from build123d import *

# Parameters (mm, degrees)
SKETCH_1_W          = 120
SKETCH_1_H          = 40
EXTRUDE_1_DEPTH     = 4.5
SKETCH_2_R          = 1.6
CUT_EXTRUDE_1_DEPTH = 127.571126249


with BuildPart() as part:
    # 草图1 → 凸台-拉伸1 (new body)
    with BuildSketch(Plane(origin=(0, 0, 0), x_dir=(1, 0, 0), z_dir=(0, 1, 0))):
        with Locations((60, 20)):
            Rectangle(SKETCH_1_W, SKETCH_1_H)
    extrude(amount=EXTRUDE_1_DEPTH)

    # 草图2 → 切除-拉伸1 (cut, through all)
    with BuildSketch(Plane.XZ):
        with Locations(Location((8, -7, 0), (0, 0, 270))):
            Circle(SKETCH_2_R)
        with Locations(Location((32, -33, 0), (0, 0, 270))):
            Circle(SKETCH_2_R)
        with Locations(Location((32, -7, 0), (0, 0, 270))):
            Circle(SKETCH_2_R)
        with Locations(Location((100, -33, 0), (0, 0, 270))):
            Circle(SKETCH_2_R)
        with Locations(Location((20, -33, 0), (0, 0, 270))):
            Circle(SKETCH_2_R)
        with Locations(Location((100, -7, 0), (0, 0, 270))):
            Circle(SKETCH_2_R)
        with Locations(Location((20, -7, 0), (0, 0, 270))):
            Circle(SKETCH_2_R)
        with Locations(Location((112, -33, 0), (0, 0, 270))):
            Circle(SKETCH_2_R)
        with Locations(Location((112, -7, 0), (0, 0, 270))):
            Circle(SKETCH_2_R)
        with Locations(Location((8, -33, 0), (0, 0, 270))):
            Circle(SKETCH_2_R)
        with Locations(Location((88, -33, 0), (0, 0, 270))):
            Circle(SKETCH_2_R)
        with Locations(Location((88, -7, 0), (0, 0, 270))):
            Circle(SKETCH_2_R)
        with BuildLine():
            Line((77, -15), (43, -15))
            ThreePointArc((43, -15), (36, -22), (43, -29))
            Line((43, -29), (77, -29))
            ThreePointArc((77, -29), (84, -22), (77, -15))
        make_face()
    extrude(amount=-CUT_EXTRUDE_1_DEPTH, mode=Mode.SUBTRACT)


solid = part.part
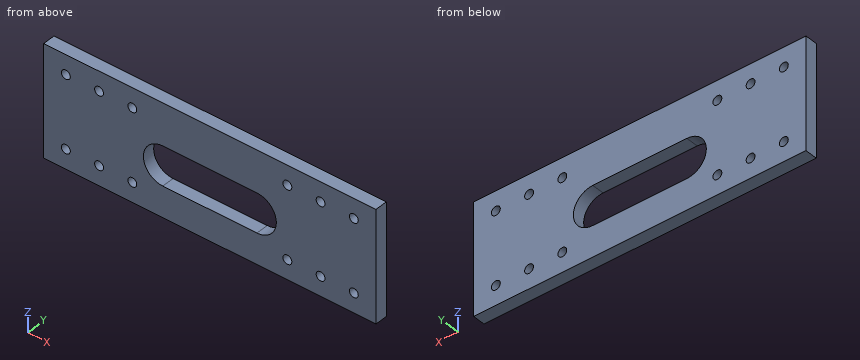
Geometry check sheet. Reference: the model listing, model coordinates, mm. Round coordinates to 2 decimals unless told otherwise and drop trailing zeros. Order: outer loops, then holes, each group sorted by start corner. A loop starts at its lowest first (then second) coordinate and runs counter-clockwise, first axis right, second up. Notation, with made-up numbers: M 15.5,-35.75 L 25.5,-35.75 A22 ccw 25.5,-13.75 Z; hole C 18.25,33.5 d4. An arc over 180 degrees is marked long. Answer in a Markdown table with one row per item. Add a question column.
Item 1: Sectioned sample at C-C, the plane x = 20. Enter the section's corners in (y, z), plus the area to 3 significant figures.
Item 2: Sectioned sample at B-B, the plane z = -33. Enter the section's corners in (x, y).
Item 3: Material ranges on L1, parallel to Z at x = 100, y = 1.3; L2, parallel to X at y = 0.9, z = -21.5; L3, parallel to Z at x = 47.5, y = 3.95, recorded low to high. Write a range as [from, to].
Item 4: Sectioned sample at A-A, the plane x = 68. Enter the section's corners in (y, z).
Item 5: Depth check by flat-ended pin: pin 1 Ø2.5 at (x, z) = (20, -7) entering from -Y. Enter the tip coordinate at first touch or a pass-through.
Item 6: Sectioned sample at D-D, the plane y = 1.2. State how many separate pieces and enclosed holes the cut face has, plus the area to 3 significant figures.
Filled in:
| question | item | result |
|---|---|---|
| 1 | outline | M 0,-40 L 4.5,-40 L 4.5,-34.6 L 0,-34.6 Z; M 0,-31.4 L 4.5,-31.4 L 4.5,-8.6 L 0,-8.6 Z; M 0,-5.4 L 4.5,-5.4 L 4.5,0 L 0,0 Z |
| 1 | area | 151 mm² |
| 2 | outline | M 0,0 L 6.4,0 L 6.4,4.5 L 0,4.5 Z; M 9.6,0 L 18.4,0 L 18.4,4.5 L 9.6,4.5 Z; M 21.6,0 L 30.4,0 L 30.4,4.5 L 21.6,4.5 Z; M 33.6,0 L 86.4,0 L 86.4,4.5 L 33.6,4.5 Z; M 89.6,0 L 98.4,0 L 98.4,4.5 L 89.6,4.5 Z; M 101.6,0 L 110.4,0 L 110.4,4.5 L 101.6,4.5 Z; M 113.6,0 L 120,0 L 120,4.5 L 113.6,4.5 Z |
| 3 | L1 | z = [-40, -34.6], [-31.4, -8.6], [-5.4, 0] |
| 3 | L2 | x = [0, 36.02], [83.98, 120] |
| 3 | L3 | z = [-40, -29], [-15, 0] |
| 4 | outline | M 0,-40 L 4.5,-40 L 4.5,-29 L 0,-29 Z; M 0,-15 L 4.5,-15 L 4.5,0 L 0,0 Z |
| 5 | pin 1 | passes through |
| 6 | separate pieces | 1 |
| 6 | enclosed holes | 13 |
| 6 | area | 4,070 mm² |
